```python
from build123d import *

# Parameters (mm, degrees)
SKETCH_1_W          = 100
SKETCH_1_H          = 60
EXTRUDE_1_DEPTH     = 1.6
SKETCH_2_R          = 1.6
CUT_EXTRUDE_1_DEPTH = 2.6
SKETCH_3_W          = 12.5
SKETCH_3_H          = 11
CUT_EXTRUDE_2_DEPTH = 2.6
FILLET_1_R          = 3
FILLET_2_R          = 1.5


with BuildPart() as part:
    # 草图1 → 凸台-拉伸1 (new body)
    with BuildSketch(Plane(origin=(0, 0, 0), x_dir=(1, 0, 0), z_dir=(0, 1, 0))):
        Rectangle(SKETCH_1_W, SKETCH_1_H)
    extrude(amount=EXTRUDE_1_DEPTH)

    # 草图2 → 切除-拉伸1 (cut, through all)
    with BuildSketch(Plane(origin=(0, 1.6, 0), x_dir=(1, 0, 0), z_dir=(0, 1, 0))):
        with Locations((-47, 27)):
            Circle(SKETCH_2_R)
        with Locations((47, 27)):
            Circle(SKETCH_2_R)
        with Locations((47, -27)):
            Circle(SKETCH_2_R)
        with Locations((-47, -27)):
            Circle(SKETCH_2_R)
    extrude(amount=-CUT_EXTRUDE_1_DEPTH, mode=Mode.SUBTRACT)

    # 草图3 → 切除-拉伸2 (cut, through all)
    with BuildSketch(Plane(origin=(0, 1.6, 0), x_dir=(1, 0, 0), z_dir=(0, 1, 0))):
        with Locations((-18.75, 24.5)):
            Rectangle(SKETCH_3_W, SKETCH_3_H)
    extrude(amount=-CUT_EXTRUDE_2_DEPTH, mode=Mode.SUBTRACT)

    # 圆角1
    fillet_1_edges = [part.edges().sort_by_distance(p)[0] for p in [
        (-50, 0.8, 30),
        (-50, 0.8, -30),
        (50, 0.8, -30),
        (50, 0.8, 30),
    ]]
    fillet(fillet_1_edges, radius=FILLET_1_R)

    # 圆角2
    fillet_2_edges = [part.edges().sort_by_distance(p)[0] for p in [
        (-25, 0.8, -19),
        (-25, 0.8, -30),
        (-12.5, 0.8, -30),
        (-12.5, 0.8, -19),
    ]]
    fillet(fillet_2_edges, radius=FILLET_2_R)


solid = part.part
```
Geometry check sheet. Reference: the model listing, model coordinates, mm. Coordinates: 2 decimals unless noted, no trailing zeros. Order: outer loops, then holes, each group sorted by start corner. A loop starts at its lowest first (then second) coordinate and runs counter-clockwise, first axis right, second up. Notation, with made-up numbers: (-13.5, 52.25) - (18.5, 52.25) arc R14 ccw to (18.5, 70.25) - close; hole circle Ø11 at (71.5, -26). An arc over 180 degrees is marked (long way). Answer in a Markdown table with one row per item. Add a question column.
1. Gauge pin test, flat ends, axial feed: pin 1 Ø4 at (x, z) = (-25, -11.5) entering from -Y; pin 2 Ø2.5 at (x, z) = (-47, 27) entering from +Y. Record the tip position at first contact, or that the pin passes through.
2. Draft check along X on faces 1 (the face through (48.526, 0.811, -27.481)), 2 (the face through (-46.14, 0.81, 25.65)), 3 (the face through (-49.14, 0.81, 29.1)), 4 (the face through (-1, 0, 0)). Enter one of: +X half, -X half, draft (parallel to the pull), parting line (faces both ways), or undercut.
3. Section check A-A (y = 0.75). Enter the section's corners in (x, z), plus the area to 3 significant figures.
4. Material ranges on L1, parallel to Z at x = -47, y = 1.05; L2, parallel to X at y = 1, z = -27; L3, parallel to X at y = 0.95, z = 27, recorded low to high. Write a range as [from, to].
Data:
| question | item | result |
|---|---|---|
| 1 | pin 1 | stops at y = 0 |
| 1 | pin 2 | passes through |
| 2 | face 1 | undercut |
| 2 | face 2 | undercut |
| 2 | face 3 | -X half |
| 2 | face 4 | draft |
| 3 | outline | (-50, -27) arc R3 ccw to (-47, -30) - (-26.5, -30) arc R1.5 ccw to (-25, -28.5) - (-25, -20.5) arc R1.5 cw to (-23.5, -19) - (-14, -19) arc R1.5 cw to (-12.5, -20.5) - (-12.5, -28.5) arc R1.5 ccw to (-11, -30) - (47, -30) arc R3 ccw to (50, -27) - (50, 27) arc R3 ccw to (47, 30) - (-47, 30) arc R3 ccw to (-50, 27) - close; hole circle Ø3.2 at (-47, -27); hole circle Ø3.2 at (-47, 27); hole circle Ø3.2 at (47, -27); hole circle Ø3.2 at (47, 27) |
| 3 | area | 5,820 mm² |
| 4 | L1 | z = [-30, -28.6], [-25.4, 25.4], [28.6, 30] |
| 4 | L2 | x = [-50, -48.6], [-45.4, -25], [-12.5, 45.4], [48.6, 50] |
| 4 | L3 | x = [-50, -48.6], [-45.4, 45.4], [48.6, 50] |
